```python
from build123d import *

# Parameters (mm, degrees)
SKETCH_1_R          = 2.1
SKETCH_1_R_2        = 1.65
SKETCH_1_R_3        = 2
SKETCH_1_R_4        = 2.05
SKETCH_1_R_5        = 9.52
EXTRUDE_1_DEPTH     = 2
SKETCH_3_W          = 52.726125437
SKETCH_3_H          = 0.98
SKETCH_3_W_2        = 46.2
SKETCH_3_H_2        = 3.817212264
EXTRUDE_2_DEPTH     = 2
SKETCH_2_R          = 2.05
SKETCH_2_W          = 32.809844138
SKETCH_2_H          = 42
CUT_EXTRUDE_1_DEPTH = 4
FILLET_1_R          = 2
FILLET_2_R          = 1.5


with BuildPart() as part:
    # 草图1 → 凸台-拉伸1 (new body)
    with BuildSketch(Plane.XY):
        with BuildLine():
            ThreePointArc((-1.457142857, 39.854285714), (-41.457142857, -0.145714286), (-1.457142857, -40.145714286))
            Line((-1.457142857, -40.145714286), (328.542857143, -40.145714286))
            ThreePointArc((328.542857143, -40.145714286), (368.542857143, -0.145714286), (328.542857143, 39.854285714))
            Line((328.542857143, 39.854285714), (-1.457142857, 39.854285714))
        make_face()
        with Locations((-1.457142857, -23.895714286)):
            Circle(SKETCH_1_R, mode=Mode.SUBTRACT)
        with Locations((-20.942714442, -11.395714286)):
            Circle(SKETCH_1_R, mode=Mode.SUBTRACT)
        with Locations((18.028428728, -11.395714286)):
            Circle(SKETCH_1_R, mode=Mode.SUBTRACT)
        with Locations((-9.957142857, -8.645714286)):
            Circle(SKETCH_1_R_2, mode=Mode.SUBTRACT)
        with Locations((7.042857143, -8.645714286)):
            Circle(SKETCH_1_R_2, mode=Mode.SUBTRACT)
        with Locations((-1.457142857, -0.145714286)):
            Circle(SKETCH_1_R_3, mode=Mode.SUBTRACT)
        with Locations((238.542857143, -16.645714286)):
            Circle(SKETCH_1_R_4, mode=Mode.SUBTRACT)
        with Locations((288.542857143, -0.145714286)):
            Circle(SKETCH_1_R_4, mode=Mode.SUBTRACT)
        with Locations((328.542857143, -0.145714286)):
            Circle(SKETCH_1_R_5, mode=Mode.SUBTRACT)
        with Locations((-9.957142857, 8.354285714)):
            Circle(SKETCH_1_R_2, mode=Mode.SUBTRACT)
        with Locations((7.042857143, 8.354285714)):
            Circle(SKETCH_1_R_2, mode=Mode.SUBTRACT)
        with Locations((-22.025246197, 11.729285714)):
            Circle(SKETCH_1_R, mode=Mode.SUBTRACT)
        with Locations((19.110960483, 11.729285714)):
            Circle(SKETCH_1_R, mode=Mode.SUBTRACT)
        with Locations((-1.457142857, 22.354285714)):
            Circle(SKETCH_1_R, mode=Mode.SUBTRACT)
        with Locations((238.542857143, 16.354285714)):
            Circle(SKETCH_1_R_4, mode=Mode.SUBTRACT)
    extrude(amount=EXTRUDE_1_DEPTH)

    # 草图3 → 凸台-拉伸2 (add)
    with BuildSketch(Plane.XY.offset(2)):
        with Locations((24.905919862, 40.344285714)):
            Rectangle(SKETCH_3_W, SKETCH_3_H)
        with Locations((18.542857143, -41.36131722)):
            Rectangle(SKETCH_3_W_2, SKETCH_3_H_2)
    extrude(amount=-EXTRUDE_2_DEPTH)

    # 草图2 → 切除-拉伸1 (cut)
    with BuildSketch(Plane.XY.offset(2)):
        with Locations((18.542857143, 33.854285714)):
            Circle(SKETCH_2_R)
        with Locations((108.542857143, 33.854285714)):
            Circle(SKETCH_2_R)
        with Locations((198.542857143, 33.854285714)):
            Circle(SKETCH_2_R)
        with Locations((288.542857143, 33.854285714)):
            Circle(SKETCH_2_R)
        with Locations((108.542857143, -34.145714286)):
            Circle(SKETCH_2_R)
        with Locations((198.542857143, -34.145714286)):
            Circle(SKETCH_2_R)
        with Locations((288.542857143, -34.145714286)):
            Circle(SKETCH_2_R)
        with Locations((18.542857143, -40.329923352)):
            Circle(SKETCH_2_R)
        Polygon((31.542857143, -21.145714286), (104.183898028, -21.145714286), (159.772133322, 20.854285714), (31.542857143, 20.854285714), align=None)
        Polygon((148.123425102, -21.145714286), (203.711660396, 20.854285714), (233.542857143, 20.854285714), (233.542857143, -21.145714286), align=None)
        with Locations((259.947779212, -0.145714286)):
            Rectangle(SKETCH_2_W, SKETCH_2_H)
        Polygon((29.492857143, -39.279923352), (37.592857143, -39.279923352), (37.592857143, -41.379923352), (37.592857143, -45.95931596), (29.492857143, -45.95931596), (29.492857143, -41.379923352), align=None)
        Polygon((-0.507142857, -39.279923352), (7.592857143, -39.279923352), (7.592857143, -41.379923352), (7.592857143, -45.95931596), (-0.507142857, -45.95931596), (-0.507142857, -41.379923352), align=None)
    extrude(amount=-CUT_EXTRUDE_1_DEPTH, mode=Mode.SUBTRACT)

    # 圆角1
    fillet_1_edges = [part.edges().sort_by_distance(p)[0] for p in [
        (243.542857143, 20.854285714, 1),
        (276.352701281, 20.854285714, 1),
        (276.352701281, -21.145714286, 1),
        (243.542857143, -21.145714286, 1),
        (31.542857143, -21.145714286, 1),
        (31.542857143, 20.854285714, 1),
        (159.772133322, 20.854285714, 1),
        (104.183898028, -21.145714286, 1),
        (203.711660396, 20.854285714, 1),
        (233.542857143, 20.854285714, 1),
        (233.542857143, -21.145714286, 1),
        (148.123425102, -21.145714286, 1),
    ]]
    fillet(fillet_1_edges, radius=FILLET_1_R)

    # 圆角2
    fillet_2_edges = [part.edges().sort_by_distance(p)[0] for p in [
        (37.592857143, -43.269923352, 1),
        (29.492857143, -43.269923352, 1),
        (7.592857143, -43.269923352, 1),
        (-0.507142857, -43.269923352, 1),
    ]]
    fillet(fillet_2_edges, radius=FILLET_2_R)


solid = part.part
```
For this review, take the finished solid that the model builds, in its own axes (mm). A direction names the side the tool comes from. Coordinates: 2 decimals unless noted, no trailing zeros. Write each loop counter-clockwise with the first axis right and the second up, starting at its lowest first coordinate (ties: lowest second). Pieces come first, ordered by that corner, then holes. Notation, with made-up numbers: (78, 0) - (127, 0) arc R25 cw to (127, 23) - close; hole circle Ø8 at (-31, 42.5). An arc over 180 degrees is marked (long way). Answer in a Markdown table with one row per item. Add a question column.
Q1. Draft analysis for pull direction X (two halves, no side actions). For faces 3 (the cylindrical face through (337.337, -3.792, 0.986)), 4 (the cylindrical face through (-41.385, 2.262, 0.986)), 5 (the flat face through (161, -1, 2)), state which applies: +X half, -X half, draft (parallel to the pull), parting line (faces both ways), or undercut.
Q2. We need section C-C, the plane x = 135. State the section outline as (y, z) points, and give its area (3 significant figures).
Q3. We need section A-A, the plane x = 264. State the section outline as (y, z) points, and give its area (3 significant figures).
Q4. Tool access review of faces 1 (the cylindrical face through (368.533, -1.025, 0.986)), 2 (the flat face through (177.7, 1.2, 1)): name each direction out of +Z, -Z, +X, -X, +Y, -Y from which nothing blocks a thin tool from reaching the whole face with its end or side.
Q5. For P1, Ø5, axis at x = -1.46, y = -0.15, coming from the -Z side; P2, Ø1, axis at y = -41, z = 1, coming from the +X side; P3, Ø0.6, axis at y = -41, z = 1, coming from the -X side; P4, Ø1, axis at x = 112.5, z = 1, coming from the -Y side, all flat-tipped, find the tip position at first contact; note any pin that passes through.
Q6. For probe 1 along X at (y, z) = (6.5, 0.7); probe 2 along X at (y, z) = (9.5, 0.95); probe 3 along Y at (x, z) = (49.5, 0.95), list the stretches that pass through material, from the lowest coordinate up.
Q7. We need section B-B, the plane z = 0.7. Count the separate pieces of the cut face and the enclosed holes in it, and give its area (3 significant figures).
Answer list:
| question | item | result |
|---|---|---|
| 1 | face 3 | undercut |
| 1 | face 4 | -X half |
| 1 | face 5 | draft |
| 2 | outline | (-40.15, 0) - (2.14, 0) - (2.14, 2) - (-40.15, 2) - close; (20.85, 0) - (39.85, 0) - (39.85, 2) - (20.85, 2) - close |
| 2 | area | 123 mm2 |
| 3 | outline | (-40.15, 0) - (-21.15, 0) - (-21.15, 2) - (-40.15, 2) - close; (20.85, 0) - (39.85, 0) - (39.85, 2) - (20.85, 2) - close |
| 3 | area | 76.0 mm2 |
| 4 | face 1 | +Z, -Z, +X |
| 4 | face 2 | +Z, -Z |
| 5 | P1 | stops at z = 0 |
| 5 | P2 | stops at x = 41.64 |
| 5 | P3 | stops at x = -4.56 |
| 5 | P4 | stops at y = -40.15 |
| 6 | probe 1 | x = -40.9 to 31.54, 140.77 to 184.71, 233.54 to 243.54, 276.35 to 321.73, 335.36 to 367.99 |
| 6 | probe 2 | x = -40.28 to -11.14, -8.77 to 5.86, 8.23 to 31.54, 144.74 to 188.68, 233.54 to 243.54, 276.35 to 367.36 |
| 6 | probe 3 | y = -40.15 to -21.15, 20.85 to 40.83 |
| 7 | separate pieces | 1 |
| 7 | enclosed holes | 26 |
| 7 | area | 23,000 mm2 |
